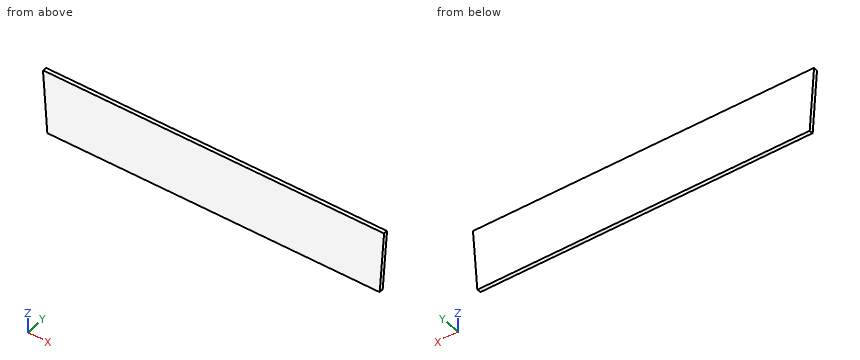
```python
from build123d import *

# Parameters (mm, degrees)
BASE_FLANGE1_DEPTH = 10
FILLET_1_0_R       = 1


# Sheet-metal steps are written as plain solids
with BuildPart() as part:
    # Sketch1 → Base-Flange1 (new body)
    with BuildSketch(Plane(origin=(0, 0, 0), x_dir=(1, 0, 0), z_dir=(0, 1, 0))):
        Polygon((-426.811710089, 160), (426.811710089, 160), (438, 0), (-438, 0), align=None)
    extrude(amount=-BASE_FLANGE1_DEPTH)

    # Fillet-1.0
    fillet_1_0_edges = [part.edges().sort_by_distance(p)[0] for p in [
        (-426.811710089, -5, -160),
        (426.811710089, -5, -160),
        (438, -5, 0),
        (-438, -5, 0),
    ]]
    fillet(fillet_1_0_edges, radius=FILLET_1_0_R)


solid = part.part
```
Check sheet for the modelled part. Datum: model origin and axes. Units: mm. Round coordinates to 2 decimals unless told otherwise and drop trailing zeros. Write each loop counter-clockwise with the first axis right and the second up, starting at its lowest first coordinate (ties: lowest second). Pieces come first, ordered by that corner, then holes. Notation, with made-up numbers: M -18.5,61.5 L 31.5,61.5 A32 cw 31.5,99.5 Z; hole C 70.5,88.25 d9. An arc over 180 degrees is marked long. Write item = value, one per line. Start each with the question number.
1. Gauge pin test, flat ends, axial feed: pin 1 (4 mm diameter, centred on y = -8, z = -136.5, fed in from -X); pin 2 (4 mm diameter, centred on y = -3.5, z = -135, fed in from +X); pin 3 (4 mm diameter, centred on y = -8, z = -94, fed in from +X). Record the tip position at first contact, or that the pin passes through.
2. Section check A-A, the plane z = -146. Record the cut outline in (x, y), then the cut area to 3 significant figures.
3. Scan lines: line 1 (X direction, y = -3, z = -17); line 2 (X direction, y = -7.75, z = -92). Record each from-to range of solid material in increasing order. Write a range as [from, to].
Results found:
q1.pin_1 = -428.59
q1.pin_2 = 428.7
q1.pin_3 = 431.57
q2.outline = M -427.79,-10 L 427.79,-10 L 427.79,0 L -427.79,0 Z
q2.area = 8,560 mm^2
q3.line_1 = [-436.81, 436.81]
q3.line_2 = [-431.57, 431.57]
